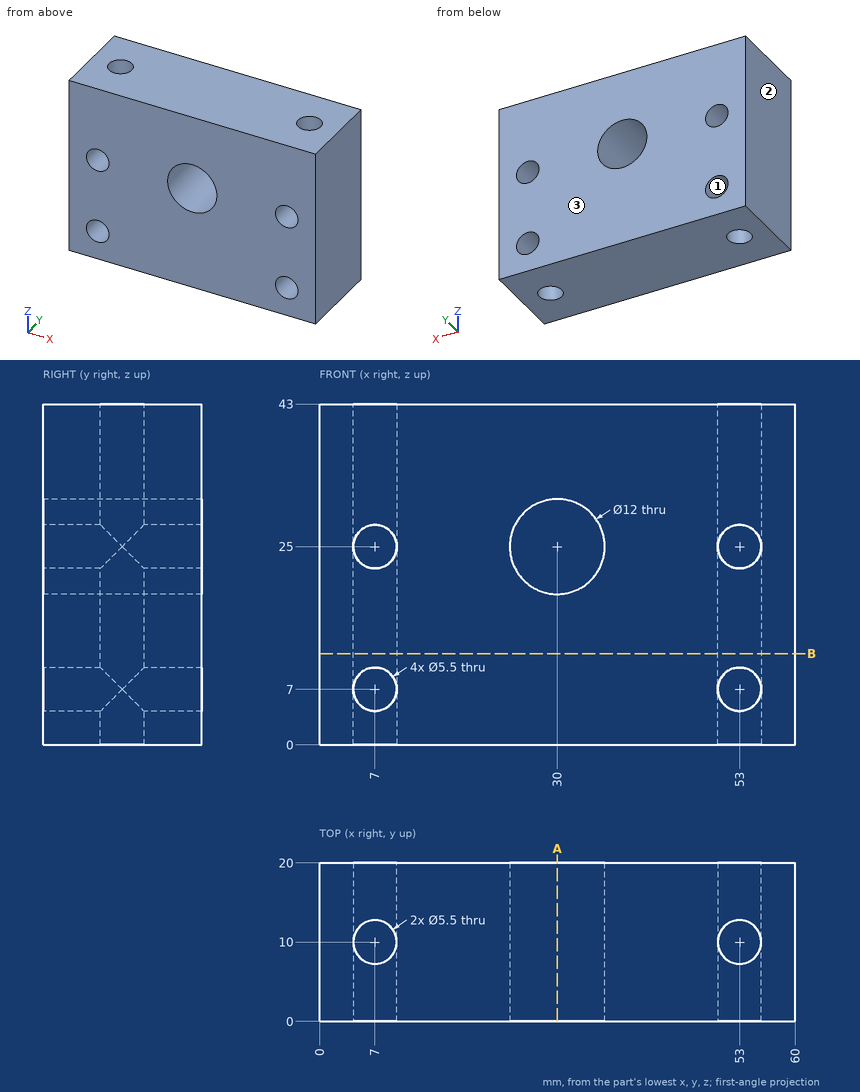
Source: three-view drawing plus pictorial views. Frame: mm from the lowest corner of the part. Give positions to 0.01 mm unless a question says otherwise; leave off trailing zeros. Write each loop counter-clockwise with the first axis right and the second up, starting at its lowest first coordinate (ties: lowest second). Pieces come first, ordered by that corner, then holes. Notation, with made-up numbers: M 12,-9.5 L 17,-9.5 A30 cw 17,21.5 Z; hole C 88.25,52.25 d7. An arc over 180 degrees is marked long. Use one line per item in the form item = value.
1. Cut plane B-B on z = 11.5. Return loops of the section in (x, y).
Outcome:
outline = M 0,0 L 60,0 L 60,20 L 0,20 Z; hole C 7,10 d5.5; hole C 53,10 d5.5
2. Cut plane A-A on x = 30. Return loops of the section in (y, z).
Outcome:
outline = M 0,0 L 20,0 L 20,19 L 0,19 Z; M 0,31 L 20,31 L 20,43 L 0,43 Z
3. Ray query, L1, parallel to X at y = 10, z = 4.5; L2, parallel to Z at x = 53, y = 5; L3, parallel to Z at x = 30, y = 14.25. Return the intervals inside material, ascending.
Outcome:
L1 = 0 to 4.25, 9.75 to 50.25, 55.75 to 60
L2 = 0 to 4.25, 9.75 to 22.25, 27.75 to 43
L3 = 0 to 19, 31 to 43
4. Mould query, pull axis X, two halves, no side actions, for the marked faces 1, 2 and 3. Classes: released by +X, released by -X, zero draft, split by the parting line, or undercut.
Outcome:
face_1 = undercut
face_2 = released by -X
face_3 = zero draft
